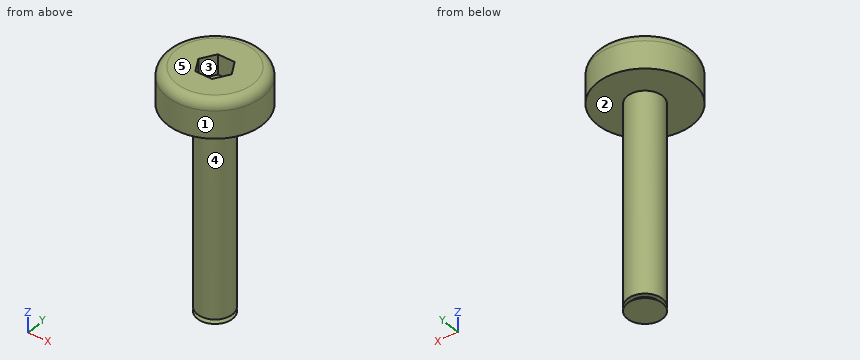
```python
from build123d import *

# Parameters (mm, degrees)
F_0045_CYLINDER_SKETCH_R    = 3.25
F_0045_CYLINDER_DEPTH       = 2.5
F_0046_FILLET_R             = 0.625
F_0047_EXTRUDE_DEPTH        = 1.385
F_0047_EXTRUDE_ROTATE_ANGLE = 120
F_0050_CYLINDER_SKETCH_R    = 1.2
F_0050_CYLINDER_DEPTH       = 13.7
F_0051_CONE_ROTATE_ANGLE    = 90


with BuildPart() as part:
    # 0045_cylinder_Sketch → 0045_cylinder (new body)
    with BuildSketch(Plane.XY):
        Circle(F_0045_CYLINDER_SKETCH_R)
    extrude(amount=F_0045_CYLINDER_DEPTH)

    # 0046_fillet
    f_0046_fillet_edges = [part.edges().sort_by_distance(p)[0] for p in [
        (-3.25, 0, 2.5),
    ]]
    fillet(f_0046_fillet_edges, radius=F_0046_FILLET_R)


with BuildPart() as body_2:
    # 0047_extrude_Sketch → 0047_extrude (new body)
    with BuildSketch(Plane.XY):
        Polygon((0, 0), (1.154700538, 0), (1.732050808, 1), (1.154700538, 2), (0, 2), (-0.577350269, 1), align=None)
    extrude(amount=F_0047_EXTRUDE_DEPTH)


with BuildPart() as body_2_1:
    # 0047_extrude_Rotate: read off the stored shape, not the designer's step
    # 0047_extrude_Rotate: moved
    add(body_2.part.rotate(Axis((0, 0, 0), (0, 0, 1)), F_0047_EXTRUDE_ROTATE_ANGLE))


with BuildPart() as body_2_2:
    # 0047_extrude_Translate: moved
    add(body_2_1.part.moved(Location((1.154700538, 0, 1.125))))


with BuildPart() as part_1:
    add(part.part)

    # 0049_sub: cut body 2
    add(body_2_2.part, mode=Mode.SUBTRACT)


with BuildPart() as body_2_2_1:
    # 0050_cylinder_Sketch → 0050_cylinder (new body)
    with BuildSketch(Plane.XY):
        Circle(F_0050_CYLINDER_SKETCH_R)
    extrude(amount=F_0050_CYLINDER_DEPTH)


with BuildPart() as body_2_2_2:
    # 0050_cylinder_Translate: moved
    add(body_2_2_1.part.moved(Location((0, 0, -13.7))))


with BuildPart() as body_3:
    # 0051_cone_Sketch → 0051_cone (revolve)
    with BuildSketch(Plane.XY, mode=Mode.PRIVATE) as f_0051_cone_sk:
        Polygon((0, 0), (1.2, 0), (0.9, 0.3), (0, 0.3), align=None)
    revolve(f_0051_cone_sk.sketch.rotate(Axis((0, -100, 0), (0, 1, 0)), 90), axis=Axis((0, -100, 0), (0, 1, 0)))


with BuildPart() as body_3_1:
    # 0051_cone_Rotate: moved
    add(body_3.part.rotate(Axis((0, 0, 0), (1, 0, 0)), F_0051_CONE_ROTATE_ANGLE))


with BuildPart() as body_3_2:
    # 0051_cone_Translate: moved
    add(body_3_1.part.moved(Location((0, 0, -14))))


with BuildPart() as body_2_2_3:
    add(body_2_2_2.part)

    # 0053_add: union body 3
    add(body_3_2.part)


with BuildPart() as part_2:
    add(part_1.part)

    # 0054_add: union body 2 2
    add(body_2_2_3.part)


solid = part_2.part
```
Part model, mm, in its own coordinate system. Face numbers are marked on the shaded views. A direction names the side the tool comes from. Give positions to 0.01 mm unless a question says otherwise; leave off trailing zeros. Order: outer loops, then holes, each group sorted by start corner. A loop starts at its lowest first (then second) coordinate and runs counter-clockwise, first axis right, second up. Notation, with made-up numbers: M -3.5,54.5 L 4.5,54.5 A10 ccw 4.5,63.5 Z; hole C 80,54.5 d8. An arc over 180 degrees is marked long. Use a Markdown table: item, result. Add a question column.
(1) Probe line 1 along Z through (x, y) = (-0.75, 2); line 2 along X through (y, z) = (0.5, -6.5); line 3 along Z through (x, y) = (2.5, 1.75). List the from-to ranges inside material, lowest first. Write a range as [from, to].
(2) Saw through at B-B, the plane x = 0. Give the cut face in (y, z) (3 decimals).
(3) Mould opens along Y. For the marked faces 3, 4 and 5 say: +Y half, -Y half, draft (parallel to the pull), parting line (faces both ways), or undercut.
(4) Drop flat-ended pins along their axis: P1, Ø1, axis at x = 0, z = -9, coming from the +Y side; P2, Ø3, axis at y = 2, z = -6.5, coming from the -X side. Give the stop position or say it passes through.
(5) 3-axis set-ups, long thin cutter, end or side, ignore diameter. For the marked faces 1 and 2: which of +Z, -Z, +X, -X, +Y, -Y reach the whole face in a straight line?
(6) Saw through at C-C, the plane z = -8.25. Give the cut face in (x, y), and give its area (3 significant figures).
(7) Saw through at A-A, the plane z = 1.5. Give the cut face in (x, y).
Answer key:
| question | item | result |
|---|---|---|
| 1 | line 1 | [0, 2.5] |
| 1 | line 2 | [-1.09, 1.09] |
| 1 | line 3 | [0, 2.33] |
| 2 | outline | M -3.25,0 L -1.2,0 L -1.2,-13.7 L -0.9,-13.7 L -1.2,-14 L 1.2,-14 L 0.9,-13.7 L 1.2,-13.7 L 1.2,0 L 3.25,0 L 3.25,1.875 A0.625 ccw 2.625,2.5 L 1,2.5 L 1,1.125 L -1,1.125 L -1,2.5 L -2.625,2.5 A0.625 ccw -3.25,1.875 Z |
| 3 | face 3 | undercut |
| 3 | face 4 | parting line |
| 3 | face 5 | draft |
| 4 | P1 | y = 1.2 |
| 4 | P2 | x = -1.09 |
| 5 | face 1 | +Z, -Z |
| 5 | face 2 | -Z |
| 6 | outline | C 0,0 d2.4 |
| 6 | area | 4.52 mm^2 |
| 7 | outline | C 0,0 d6.5; hole M -1.15,0 L -0.58,-1 L 0.58,-1 L 1.15,0 L 0.58,1 L -0.58,1 Z |
